Could you check a few things on this model? Use its own coordinates, in mm. A direction names the side the tool comes from. Round coordinates to 2 decimals unless told otherwise and drop trailing zeros. Order: outer loops, then holes, each group sorted by start corner. A loop starts at its lowest first (then second) coordinate and runs counter-clockwise, first axis right, second up. Notation, with made-up numbers: (88.5, 20) -> (121.5, 20) arc R8 cw to (121.5, 35) -> close; hole circle Ø8 at (60.25, -17.75). An arc over 180 degrees is marked (long way). One line per question, with ' | ' between items.
```python
from build123d import *

# Parameters (mm, degrees)
SKETCH_1_R      = 3.555
SKETCH_1_R_2    = 2.5
EXTRUDE_1_DEPTH = 6
EXTRUDE_START   = 2.5
SKETCH_1_3_R    = 3.555
SKETCH_1_3_R_2  = 2.5
EXTRUDE_2_DEPTH = 2.5


with BuildPart() as part:
    # Sketch 1 → Extrude 1 (new body)
    # profile 1 of 2: a face of its own
    with BuildSketch(Plane(origin=(0, 0, 0), x_dir=(1, 0, 0), z_dir=(0, 1, 0))):
        Polygon((-0.928202951, -7.442501227), (1.958548395, -2.442501227), (-0.928202951, 2.557498773), (-6.701705643, 2.557498773), (-9.588456989, -2.442501227), (-6.701705643, -7.442501227), align=None)
        with Locations((-3.814954297, -2.442501227)):
            Circle(SKETCH_1_R, mode=Mode.SUBTRACT)
    # profile 2 of 2: a face of its own
    with BuildSketch(Plane(origin=(0, 0, 0), x_dir=(1, 0, 0), z_dir=(0, 1, 0))):
        with Locations((-3.814954297, -2.442501227)):
            Circle(SKETCH_1_R)
        with Locations(Location((-3.024954297, -2.442501227, 0), (0, 0, 270))):
            Circle(SKETCH_1_R_2, mode=Mode.SUBTRACT)
    extrude(amount=-EXTRUDE_1_DEPTH)

    # Sketch 1_3 → Extrude 2 (add)
    with BuildSketch(Plane(origin=(0, 0, 0), x_dir=(1, 0, 0), z_dir=(0, 1, 0)).offset(EXTRUDE_START)):
        with Locations(Location((-3.814954297, -2.442501227, 0), (0, 0, 270))):
            Circle(SKETCH_1_3_R)
        with Locations(Location((-3.024954297, -2.442501227, 0), (0, 0, 270))):
            Circle(SKETCH_1_3_R_2, mode=Mode.SUBTRACT)
    extrude(amount=-EXTRUDE_2_DEPTH)


solid = part.part
```
1. If we mould it in two halves opening along Z, with no side actions, what happens to faces 3 (the face through (-0.29, 1.27, 1.98)), 4 (the face through (-0.92, -1.69, 3.79)), 5 (the face through (0.535, -2.958, -0.022))? For each: pulls with the +Z half, pulls with the -Z half, needs draft (parallel to the pull), parting line crosses it, or undercut.
From the geometry:
face 3: parting line crosses it | face 4: undercut | face 5: pulls with the -Z half
2. On a 3-axis mill with a long thin cutter (end or side, diameter ignored), from which of +Z, -Z, +X, -X, +Y, -Y can I reach the whole of each face in a straight line? I mean faces 1 (the face through (-4, -3, -2.557)), 2 (the face through (0, 0, 2)). Say none if no direction works.
From the geometry:
face 1: -Z, +X, -X, +Y, -Y | face 2: +Y
3. I want a section at A-A on z = 2. List the corners of the cut face in (x, y) for me.
From the geometry:
outline: (-9.33, -6) -> (-5.49, -6) -> (-5.49, 2.5) -> (-7.34, 2.5) -> (-7.34, 0) -> (-9.33, 0) -> close; (-0.56, -6) -> (1.7, -6) -> (1.7, 0) -> (-0.29, 0) -> (-0.29, 2.5) -> (-0.56, 2.5) -> close
4. I need wall thicknesses on probe 1 along X at (y, z) = (-1.75, 2); probe 2 along X at (y, z) = (-1.5, 1); probe 3 along Y at (x, z) = (-9, 2.25). Which ranges of each line are inside material? Lowest first, please.
From the geometry:
probe 1: x = -9.33 to -5.49, -0.56 to 1.7 | probe 2: x = -8.76 to -5.07, -0.98 to 1.13 | probe 3: y = -6 to 0
5. I want a section at D-D on z = -1.5. List the corners of the cut face in (x, y) for me, and give its area (3 significant figures).
From the geometry:
outline: (-7.31, -6) -> (-0.32, -6) -> (-0.32, 0) -> (-7.31, 0) -> close | area: 42.0 mm²
6. I want a section at C-C on y = -4.75. List the corners of the cut face in (x, z) for me, and give its area (3 significant figures).
From the geometry:
outline: (-9.59, 2.44) -> (-6.7, -2.56) -> (-0.93, -2.56) -> (1.96, 2.44) -> (-0.93, 7.44) -> (-6.7, 7.44) -> close; hole circle Ø5 at (-3.02, 2.44) | area: 67.0 mm²
7. I'm going to push flat-ended pins straight in: pin 1 (1.5 mm diameter, centred on x = 0.5, y = -2, fed in from +Z); pin 2 (1.5 mm diameter, centred on y = -3.5, z = 0, fed in from +X); pin 3 (3 mm diameter, centred on y = -2, z = 5, fed in from -X). Where does each tip first touch, or does it pass through?
From the geometry:
pin 1: stops at z = 6.27 | pin 2: stops at x = 0.98 | pin 3: stops at x = -8.98
8. I want a section at B-B on x = -3.25. List the corners of the cut face in (y, z) for me, and give its area (3 significant figures).
From the geometry:
outline: (-6, -2.56) -> (0, -2.56) -> (0, -1.07) -> (2.5, -1.07) -> (2.5, -0.05) -> (-6, -0.05) -> close; (-6, 4.93) -> (2.5, 4.93) -> (2.5, 5.95) -> (0, 5.95) -> (0, 7.44) -> (-6, 7.44) -> close | area: 35.2 mm²
